The listing builds one solid part. Answer for the finished solid, in the listing's coordinates (mm). Coordinates: 2 decimals unless noted, no trailing zeros. Return JSON: item names as keys, results as strings. Group by question number.
1. Find the intervals of material crossed by line 1 along Y through (x, z) = (-494.5, -13.25); line 2 along Z through (x, y) = (-751, -14.05); line 3 along Z through (x, y) = (736, -13.15), in increasing order.
2. Section A-A (x = 471.5) is taken. State how many separate pieces and enclosed holes the cut face has, and give its area (3 significant figures).
3. Each of these flat-tipped pins is pushed along its axis until it touches: P1, Ø1.5, axis at y = 9, z = 11.5, coming from the +X side; P2, Ø1.5, axis at y = 10, z = 4.5, coming from the +X side. Where does it stop, or does it pass through?
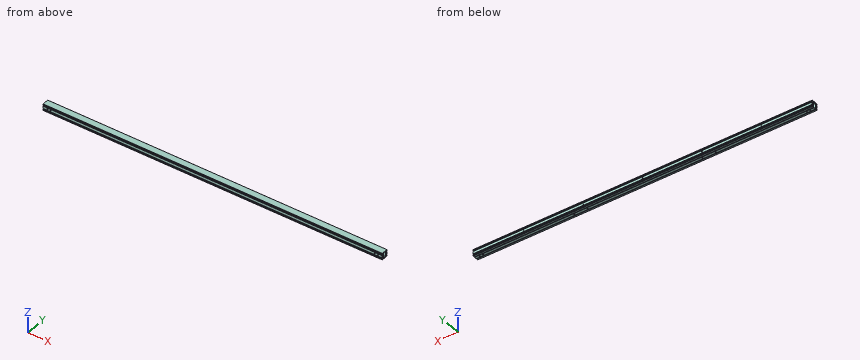
```python
from build123d import *

# Parameters (mm, degrees)
SKETCH_1_W             = 23.5
SKETCH_1_H             = 12
EXTRUDE_1_DEPTH        = 771
HOLE_WIZARD_M6_1_D     = 5
HOLE_WIZARD_M6_1_DEPTH = 15
HOLE_WIZARD_M6_1_TIP   = 1.502151548
HOLE_WIZARD_M6_2_D     = 5
HOLE_WIZARD_M6_2_DEPTH = 15
HOLE_WIZARD_M6_2_TIP   = 1.502151548
HOLE_WIZARD_M4_1_D     = 3.3
HOLE_WIZARD_M4_1_DEPTH = 10.1
HOLE_WIZARD_M4_1_TIP   = 0.991420021
HOLE_WIZARD_M6_3_D     = 5
HOLE_WIZARD_M6_3_DEPTH = 15
HOLE_WIZARD_M6_3_TIP   = 1.502151548


with BuildPart() as part:
    # 草图1 → 凸台-拉伸1 (new, symmetric)
    with BuildSketch(Plane(origin=(0, 0, 0), x_dir=(0, 0, -1), z_dir=(1, 0, 0))):
        with BuildLine():
            Line((-14, 15), (-11.5, 15))
            Line((-11.5, 15), (-11.5, 13.5))
            Line((-11.5, 13.5), (-11.4, 13.5))
            ThreePointArc((-11.4, 13.5), (-11.117157288, 13.382842712), (-11, 13.1))
            Line((-11, 13.1), (-11, 12))
            Line((-11, 12), (-9.5, 12))
            Line((-9.5, 12), (-9.5, 15))
            Line((-9.5, 15), (-8, 15))
            Line((-8, 15), (-8, 12.5))
            Line((-8, 12.5), (-5, 12.5))
            Line((-5, 12.5), (-5, 15))
            Line((-5, 15), (5, 15))
            Line((5, 15), (5, 12.5))
            Line((5, 12.5), (8, 12.5))
            Line((8, 12.5), (8, 15))
            Line((8, 15), (9.5, 15))
            Line((9.5, 15), (9.5, 12))
            Line((9.5, 12), (11, 12))
            Line((11, 12), (11, 13.1))
            ThreePointArc((11, 13.1), (11.117157288, 13.382842712), (11.4, 13.5))
            Line((11.4, 13.5), (11.5, 13.5))
            Line((11.5, 13.5), (11.5, 15))
            Line((11.5, 15), (14, 15))
            ThreePointArc((14, 15), (14.707106781, 14.707106781), (15, 14))
            Line((15, 14), (15, 8))
            Line((15, 8), (12.5, 8))
            Line((12.5, 8), (12.5, 5))
            Line((12.5, 5), (15, 5))
            Line((15, 5), (15, -5))
            Line((15, -5), (12.5, -5))
            Line((12.5, -5), (12.5, -8))
            Line((12.5, -8), (15, -8))
            Line((15, -8), (15, -14))
            ThreePointArc((15, -14), (14.707106781, -14.707106781), (14, -15))
            Line((14, -15), (11.5, -15))
            Line((11.5, -15), (11.5, -13.5))
            Line((11.5, -13.5), (11.4, -13.5))
            ThreePointArc((11.4, -13.5), (11.117157288, -13.382842712), (11, -13.1))
            Line((11, -13.1), (11, -12))
            Line((11, -12), (9.5, -12))
            Line((9.5, -12), (9.5, -15))
            Line((9.5, -15), (8, -15))
            Line((8, -15), (8, -12.5))
            Line((8, -12.5), (5, -12.5))
            Line((5, -12.5), (5, -15))
            Line((5, -15), (-5, -15))
            Line((-5, -15), (-5, -12.5))
            Line((-5, -12.5), (-8, -12.5))
            Line((-8, -12.5), (-8, -15))
            Line((-8, -15), (-9.5, -15))
            Line((-9.5, -15), (-9.5, -12))
            Line((-9.5, -12), (-11, -12))
            Line((-11, -12), (-11, -13.1))
            ThreePointArc((-11, -13.1), (-11.117157288, -13.382842712), (-11.4, -13.5))
            Line((-11.4, -13.5), (-11.5, -13.5))
            Line((-11.5, -13.5), (-11.5, -15))
            Line((-11.5, -15), (-14, -15))
            ThreePointArc((-14, -15), (-14.707106781, -14.707106781), (-15, -14))
            Line((-15, -14), (-15, 14))
            ThreePointArc((-15, 14), (-14.707106781, 14.707106781), (-14, 15))
        make_face()
        with BuildLine():
            Line((12, -10.5), (12, -8.5))
            ThreePointArc((12, -8.5), (11.853553391, -8.146446609), (11.5, -8))
            Line((11.5, -8), (-11.5, -8))
            ThreePointArc((-11.5, -8), (-11.853553391, -8.146446609), (-12, -8.5))
            Line((-12, -8.5), (-12, -10.5))
            ThreePointArc((-12, -10.5), (-11.853553391, -10.853553391), (-11.5, -11))
            Line((-11.5, -11), (11.5, -11))
            ThreePointArc((11.5, -11), (11.853553391, -10.853553391), (12, -10.5))
        make_face(mode=Mode.SUBTRACT)
        with BuildLine():
            Line((-11.5, 11), (11.5, 11))
            ThreePointArc((11.5, 11), (11.853553391, 10.853553391), (12, 10.5))
            Line((12, 10.5), (12, 8.5))
            ThreePointArc((12, 8.5), (11.853553391, 8.146446609), (11.5, 8))
            Line((11.5, 8), (-11.5, 8))
            ThreePointArc((-11.5, 8), (-11.853553391, 8.146446609), (-12, 8.5))
            Line((-12, 8.5), (-12, 10.5))
            ThreePointArc((-12, 10.5), (-11.853553391, 10.853553391), (-11.5, 11))
        make_face(mode=Mode.SUBTRACT)
        Rectangle(SKETCH_1_W, SKETCH_1_H, mode=Mode.SUBTRACT)
    extrude(amount=EXTRUDE_1_DEPTH, both=True)

    # M6 螺纹孔1
    with Locations(Plane.XZ.offset(15)):
        with Locations((-751, 0), (-736, 0), (736, 0), (751, 0)):
            Hole(HOLE_WIZARD_M6_1_D / 2, depth=HOLE_WIZARD_M6_1_DEPTH)
            with Locations((0, 0, -(HOLE_WIZARD_M6_1_DEPTH + HOLE_WIZARD_M6_1_TIP / 2))):  # 118° drill point
                Cone(0, HOLE_WIZARD_M6_1_D / 2, HOLE_WIZARD_M6_1_TIP, mode=Mode.SUBTRACT)

    # M6 螺纹孔2
    with Locations(Plane(origin=(0, 0, -15), x_dir=(-1, 0, 0), z_dir=(0, 0, -1))):
        with Locations((-751, 0), (-736, 0), (736, 0), (751, 0)):
            Hole(HOLE_WIZARD_M6_2_D / 2, depth=HOLE_WIZARD_M6_2_DEPTH)
            with Locations((0, 0, -(HOLE_WIZARD_M6_2_DEPTH + HOLE_WIZARD_M6_2_TIP / 2))):  # 118° drill point
                Cone(0, HOLE_WIZARD_M6_2_D / 2, HOLE_WIZARD_M6_2_TIP, mode=Mode.SUBTRACT)

    # M4 螺纹孔1
    with Locations(Plane(origin=(0, 15, 0), x_dir=(-1, 0, 0), z_dir=(0, 1, 0))):
        with Locations((-540, 0), (-270, 0), (0, 0), (270, 0), (540, 0)):
            Hole(HOLE_WIZARD_M4_1_D / 2, depth=HOLE_WIZARD_M4_1_DEPTH)
            with Locations((0, 0, -(HOLE_WIZARD_M4_1_DEPTH + HOLE_WIZARD_M4_1_TIP / 2))):  # 118° drill point
                Cone(0, HOLE_WIZARD_M4_1_D / 2, HOLE_WIZARD_M4_1_TIP, mode=Mode.SUBTRACT)

    # M6 螺纹孔3
    with Locations(Plane(origin=(0, 0, -15), x_dir=(-1, 0, 0), z_dir=(0, 0, -1))):
        with Locations((321, 0), (261, 0), (-261, 0), (-321, 0)):
            Hole(HOLE_WIZARD_M6_3_D / 2, depth=HOLE_WIZARD_M6_3_DEPTH)
            with Locations((0, 0, -(HOLE_WIZARD_M6_3_DEPTH + HOLE_WIZARD_M6_3_TIP / 2))):  # 118° drill point
                Cone(0, HOLE_WIZARD_M6_3_D / 2, HOLE_WIZARD_M6_3_TIP, mode=Mode.SUBTRACT)


solid = part.part
```
The answers:
{
 "1": {"line 1": "y = -15 to -8, -5 to 5, 8 to 15", "line 2": "z = -15 to -11.5, -9.5 to -8, -5 to -2.5, 2.5 to 5, 8 to 9.5, 11.5 to 15", "line 3": "z = -15 to -11, -9.5 to -8, -5 to -2.5, 2.5 to 5, 8 to 9.5, 11 to 15"},
 "2": {"separate pieces": "1", "enclosed holes": "3", "area": "407 mm2"},
 "3": {"P1": "stops at x = 771", "P2": "passes through"}
}
